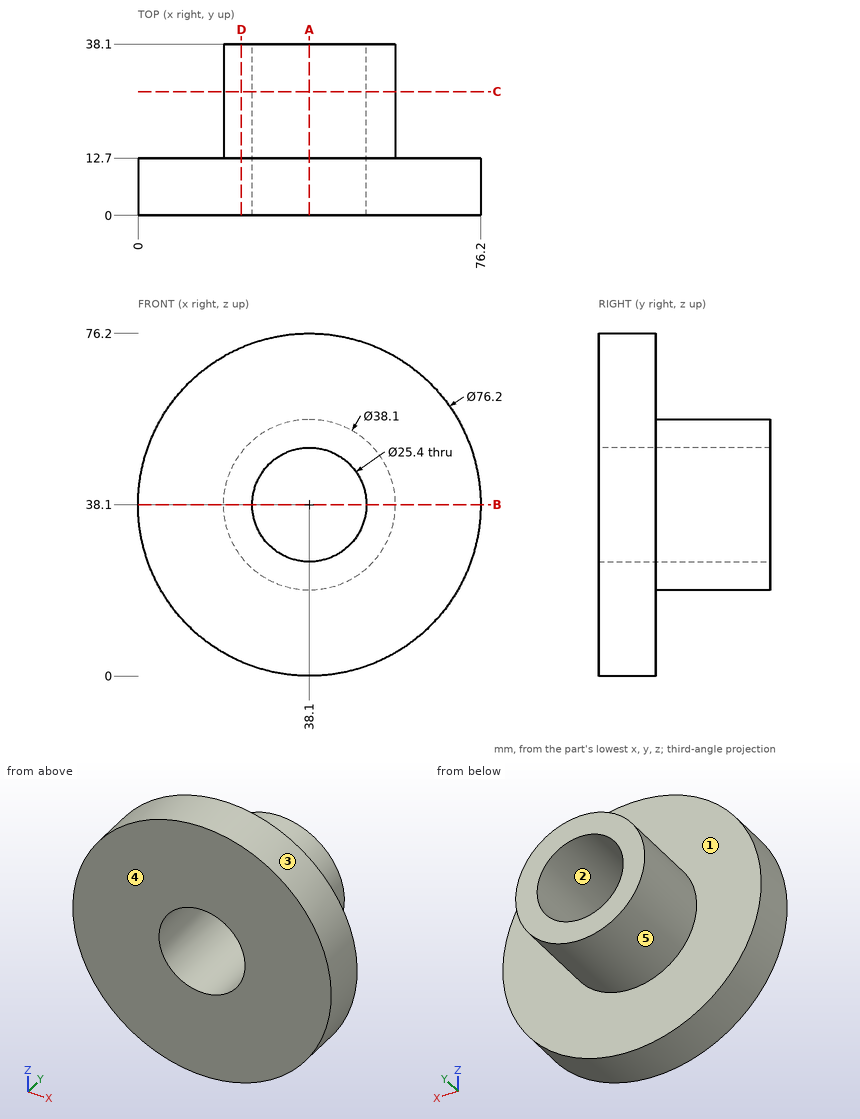
Design review of the part shown in the three views and the two pictorial views. Dimensions are in mm from the part's minimum x, y and z. A direction names the side the tool comes from. Give positions to 0.01 mm unless a question says otherwise; leave off trailing zeros. Loops run counter-clockwise (first coordinate to the right, second up) from the corner with the lowest first, then second, coordinate; pieces in that order, holes last. Notation, with made-up numbers: (70.25, 48) -> (110.25, 48) arc R22 cw to (110.25, 74) -> close; hole circle Ø6 at (11, -14). An arc over 180 degrees is marked (long way). One line per question, with ' | ' between items.
1) We need section B-B (z = 38.1). Write out the cut boundary in (x, y), plus the area to 3 significant figures.
Resolved:
outline: (0, 0) -> (25.4, 0) -> (25.4, 38.1) -> (19.05, 38.1) -> (19.05, 12.7) -> (0, 12.7) -> close; (50.8, 0) -> (76.2, 0) -> (76.2, 12.7) -> (57.15, 12.7) -> (57.15, 38.1) -> (50.8, 38.1) -> close | area: 968 mm2
2) The part is to be moulded in two halves that separate along Z. For the marked faces 1, 2 and 3, say which applies: +Z half, -Z half, draft (parallel to the pull), parting line (faces both ways), or undercut.
Resolved:
face 1: draft | face 2: undercut | face 3: parting line
3) We need section A-A (x = 38.1). Write out the cut boundary in (y, z), plus the area to 3 significant figures.
Resolved:
outline: (0, 0) -> (12.7, 0) -> (12.7, 19.05) -> (38.1, 19.05) -> (38.1, 25.4) -> (0, 25.4) -> close; (0, 50.8) -> (38.1, 50.8) -> (38.1, 57.15) -> (12.7, 57.15) -> (12.7, 76.2) -> (0, 76.2) -> close | area: 968 mm2
4) To check wall thickness, follow probe 1 along X at (y, z) = (9, 38.1); probe 2 along X at (y, z) = (29, 38); probe 3 along Y at (x, z) = (66, 28). State the ranges of each line that lie inside material, in increasing order.
Resolved:
probe 1: x = 0 to 25.4, 50.8 to 76.2 | probe 2: x = 19.05 to 25.4, 50.8 to 57.15 | probe 3: y = 0 to 12.7
5) We need section C-C (y = 27.5). Write out the cut boundary in (x, z), plus the area to 3 significant figures.
Resolved:
outline: circle Ø38.1 at (38.1, 38.1); hole circle Ø25.4 at (38.1, 38.1) | area: 633 mm2
6) We need section D-D (x = 23). Write out the cut boundary in (y, z), plus the area to 3 significant figures.
Resolved:
outline: (0, 3.12) -> (12.7, 3.12) -> (12.7, 26.49) -> (38.1, 26.49) -> (38.1, 49.71) -> (12.7, 49.71) -> (12.7, 73.08) -> (0, 73.08) -> close | area: 1,480 mm2
7) For the marked faces 4 and 5, list the 3-axis set-ups (+Z, -Z, +X, -X, +Y, -Y) from which the entire face can be reached by the end or side of a thin tool; tool diameter is ignored.
Resolved:
face 4: +Z, -Z, +X, -X, -Y | face 5: +Y
8) Insertion check: pin 1 Ø8 at (x, z) = (55.5, 55.5) entering from +Y; pin 2 Ø10 at (x, y) = (56.5, 27) entering from +Z; pin 3 Ø1.5 at (x, y) = (32, 12.5) entering from +Z. Each pin has a flat end and moves straight along its axis. Give the tip position at first contact, or say it passes through.
Resolved:
pin 1: stops at y = 12.7 | pin 2: stops at z = 51.64 | pin 3: stops at z = 75.82
